Read the model definition and answer for the solid it produces. Units are mm, in the model's axes. A direction names the side the tool comes from. Coordinates: 2 decimals unless noted, no trailing zeros. Write each loop counter-clockwise with the first axis right and the second up, starting at its lowest first coordinate (ties: lowest second). Pieces come first, ordered by that corner, then holes.
Item 1: Each of these flat-tipped pins is pushed along its axis until it touches: P1, Ø8, axis at x = -0.5, z = 60, coming from the +Y side; P2, Ø4, axis at x = 0, y = 0, coming from the -Z side; P3, Ø3, axis at x = -5, y = -6, coming from the +Z side; P4, Ø4, axis at x = 0, z = 68, coming from the -Y side. Where does it stop, or does it pass through?
Item 2: Section A-A (y = 0) is taken. Give the vertices of the cut face in (x, z).
Item 3: Straight lines are drawn through the part: probe 1 along X at (y, z) = (0, 70); probe 2 along Y at (x, z) = (4.25, 83.5). For each, find the intervals that lie inside material, in ascending order.
Item 4: A tool of negligible diameter and unlimited length cuts with its end or side. For faces 1 (the face through (0, -3.6, 77)), 2 (the face through (4, -8.2, 77)), 3 (the face through (0, 3.6, 77)), 4 (the face through (-6, 10, 77)), 5 (the face through (10, -6, 77)), from which of +Z, -Z, +X, -X, +Y, -Y can it reach the whole face along a straight path? Write none if from no direction.
Item 5: Determine the mould class of faces 6 (the face through (10, 6, 77)), 7 (the face through (-8.2, 4, 77)), 8 (the face through (-10, -6, 77)) for opening direction X: released by +X, released by -X, zero draft, split by the parting line, or undercut.
from build123d import *

# Parameters (mm, degrees)
SKETCH1_R           = 2.1
BOSS_EXTRUDE1_DEPTH = 155.6
CUT_EXTRUDE1_DEPTH  = 66


with BuildPart() as part:
    # Sketch1 → Boss-Extrude1 (new body)
    with BuildSketch(Plane.XY):
        with BuildLine():
            Line((-4.9, -10), (-3.1, -8.2))
            Line((-3.1, -8.2), (-5.5, -8.2))
            Line((-5.5, -8.2), (-5.5, -6.560660172))
            Line((-5.5, -6.560660172), (-2.539339828, -3.6))
            Line((-2.539339828, -3.6), (2.539339828, -3.6))
            Line((2.539339828, -3.6), (5.5, -6.560660172))
            Line((5.5, -6.560660172), (5.5, -8.2))
            Line((5.5, -8.2), (3.1, -8.2))
            Line((3.1, -8.2), (4.9, -10))
            Line((4.9, -10), (8, -10))
            ThreePointArc((8, -10), (9.414213562, -9.414213562), (10, -8))
            Line((10, -8), (10, -4.9))
            Line((10, -4.9), (8.2, -3.1))
            Line((8.2, -3.1), (8.2, -5.5))
            Line((8.2, -5.5), (6.560660172, -5.5))
            Line((6.560660172, -5.5), (3.6, -2.539339828))
            Line((3.6, -2.539339828), (3.6, 2.539339828))
            Line((3.6, 2.539339828), (6.560660172, 5.5))
            Line((6.560660172, 5.5), (8.2, 5.5))
            Line((8.2, 5.5), (8.2, 3.1))
            Line((8.2, 3.1), (10, 4.9))
            Line((10, 4.9), (10, 8))
            ThreePointArc((10, 8), (9.414213562, 9.414213562), (8, 10))
            Line((8, 10), (4.9, 10))
            Line((4.9, 10), (3.1, 8.2))
            Line((3.1, 8.2), (5.5, 8.2))
            Line((5.5, 8.2), (5.5, 6.560660172))
            Line((5.5, 6.560660172), (2.539339828, 3.6))
            Line((2.539339828, 3.6), (-2.539339828, 3.6))
            Line((-2.539339828, 3.6), (-5.5, 6.560660172))
            Line((-5.5, 6.560660172), (-5.5, 8.2))
            Line((-5.5, 8.2), (-3.1, 8.2))
            Line((-3.1, 8.2), (-4.9, 10))
            Line((-4.9, 10), (-8, 10))
            ThreePointArc((-8, 10), (-9.414213562, 9.414213562), (-10, 8))
            Line((-10, 8), (-10, 4.9))
            Line((-10, 4.9), (-8.2, 3.1))
            Line((-8.2, 3.1), (-8.2, 5.5))
            Line((-8.2, 5.5), (-6.560660172, 5.5))
            Line((-6.560660172, 5.5), (-3.6, 2.539339828))
            Line((-3.6, 2.539339828), (-3.6, -2.539339828))
            Line((-3.6, -2.539339828), (-6.560660172, -5.5))
            Line((-6.560660172, -5.5), (-8.2, -5.5))
            Line((-8.2, -5.5), (-8.2, -3.1))
            Line((-8.2, -3.1), (-10, -4.9))
            Line((-10, -4.9), (-10, -8))
            ThreePointArc((-10, -8), (-9.414213562, -9.414213562), (-8, -10))
            Line((-8, -10), (-4.9, -10))
        make_face()
        Circle(SKETCH1_R, mode=Mode.SUBTRACT)
    extrude(amount=BOSS_EXTRUDE1_DEPTH)

    # Sketch2 → Cut-Extrude1 (cut)
    with BuildSketch(Plane.ZY.offset(10)):
        Polygon((155.6, 10), (135.6, -10), (155.6, -10), align=None)
        Polygon((0, 10), (20, -10), (0, -10), align=None)
    extrude(amount=-CUT_EXTRUDE1_DEPTH, mode=Mode.SUBTRACT)


solid = part.part
Established:
1. P1: stops at y = 9.6
1. P2: passes through
1. P3: stops at z = 141.1
1. P4: stops at y = -3.6
2. outline: (-3.6, 10) - (-2.1, 10) - (-2.1, 145.6) - (-3.6, 145.6) - close; (2.1, 10) - (3.6, 10) - (3.6, 145.6) - (2.1, 145.6) - close
3. probe 1: x = -3.6 to -2.1, 2.1 to 3.6
3. probe 2: y = -9.35 to -8.2, -5.31 to -3.19, 3.19 to 5.31, 8.2 to 9.35
4. face 1: +Z, -Z, -Y
4. face 2: +Z, -Z
4. face 3: +Z, -Z, +Y
4. face 4: +Z, -Z, +X, -X, +Y
4. face 5: +Z, -Z, +X, +Y, -Y
5. face 6: released by +X
5. face 7: undercut
5. face 8: released by -X
